CAD build for the part. Positions are in the model's coordinates, mm. A direction names the side the tool comes from. Coordinates: 2 decimals unless noted, no trailing zeros. Write each loop counter-clockwise with the first axis right and the second up, starting at its lowest first coordinate (ties: lowest second). Pieces come first, ordered by that corner, then holes.
```python
from build123d import *

# Parameters (mm, degrees)
F0_R     = 12.2
F0_R_2   = 6.5
F1_DEPTH = 1
F3_W     = 5.6
F3_H     = 3.1
F3_W_2   = 3.1
F3_H_2   = 5.6
F4_DEPTH = 1.1


with BuildPart() as f1:
    # F0 (on Top) → F1 (new body)
    with BuildSketch(Plane.XY):
        Circle(F0_R)
        Circle(F0_R_2, mode=Mode.SUBTRACT)
    extrude(amount=F1_DEPTH)

    # F3 (on offset) → F4 (join)
    with BuildSketch(Plane.XY.offset(1)):
        with Locations((0, 9)):
            Rectangle(F3_W, F3_H)
        with Locations((9, 0)):
            Rectangle(F3_W_2, F3_H_2)
        with Locations((0, -9)):
            Rectangle(F3_W, F3_H)
        with Locations((-9, 0)):
            Rectangle(F3_W_2, F3_H_2)
    extrude(amount=F4_DEPTH)


solid = f1.part
```
Item 1: Saw through at B-B, the plane x = 0. Write the cut outline in (y, z), and give its area (3 significant figures).
Item 2: Flat gauge pins, fed straight in: pin 1 Ø0.9 at (y, z) = (9.5, 1.5) entering from -X; pin 2 Ø6 at (x, y) = (-5.5, 6) entering from +Z; pin 3 Ø1.2 at (y, z) = (-8.5, 2) entering from +X; pin 4 Ø5 at (x, y) = (2, 0) entering from -Z. Where does each tip first touch, or does it go through?
Item 3: Wall check: line 1 along Y through (x, z) = (0, 0.6); line 2 along Y through (x, z) = (0, 1.25); line 3 along Z through (x, y) = (-3.25, -11). Give the ranges that are in metal, low to high.
Item 4: Two-plate mould, pull along X, no slides. Class faces 5 (the cylindrical face through (-5.158, -3.955, 0.493)), 6 (the flat face through (9, 2.8, 1.5)), 7 (the flat face through (2.8, -9, 1.5)): +X half, -X half, draft (parallel to the pull), parting line (faces both ways), or undercut.
Item 5: Saw through at D-D, the plane y = -8. Write the cut outline in (x, z).
Item 6: Which spindle directions (+Z, -Z, +X, -X, +Y, -Y) get a long thin tool onto all of the face, cutting with end or side? Do faces 1 (the flat face through (-2.8, 9, 1.5)), 2 (the flat face through (10.55, 0, 1.5)), 3 (the flat face through (0, 7.45, 1.5)), 4 (the flat face through (-9, -2.8, 1.5)). Say none if no direction does.
Item 7: Saw through at A-A, the plane z = 1.65. Write the cut outline in (x, y).
Working result:
1. outline: (-12.2, 0) - (-6.5, 0) - (-6.5, 1) - (-7.45, 1) - (-7.45, 2.1) - (-10.55, 2.1) - (-10.55, 1) - (-12.2, 1) - close; (6.5, 0) - (12.2, 0) - (12.2, 1) - (10.55, 1) - (10.55, 2.1) - (7.45, 2.1) - (7.45, 1) - (6.5, 1) - close
1. area: 18.2 mm2
2. pin 1: stops at x = -2.8
2. pin 2: stops at z = 1
2. pin 3: stops at x = 2.8
2. pin 4: passes through
3. line 1: y = -12.2 to -6.5, 6.5 to 12.2
3. line 2: y = -10.55 to -7.45, 7.45 to 10.55
3. line 3: z = 0 to 1
4. face 5: undercut
4. face 6: draft
4. face 7: +X half
5. outline: (-9.21, 0) - (9.21, 0) - (9.21, 1) - (2.8, 1) - (2.8, 2.1) - (-2.8, 2.1) - (-2.8, 1) - (-9.21, 1) - close
6. face 1: +Z, -X, +Y, -Y
6. face 2: +Z, +X, +Y, -Y
6. face 3: +Z, +X, -X
6. face 4: +Z, +X, -X, -Y
7. outline: (-10.55, -2.8) - (-7.45, -2.8) - (-7.45, 2.8) - (-10.55, 2.8) - close; (-2.8, -10.55) - (2.8, -10.55) - (2.8, -7.45) - (-2.8, -7.45) - close; (-2.8, 7.45) - (2.8, 7.45) - (2.8, 10.55) - (-2.8, 10.55) - close; (7.45, -2.8) - (10.55, -2.8) - (10.55, 2.8) - (7.45, 2.8) - close
